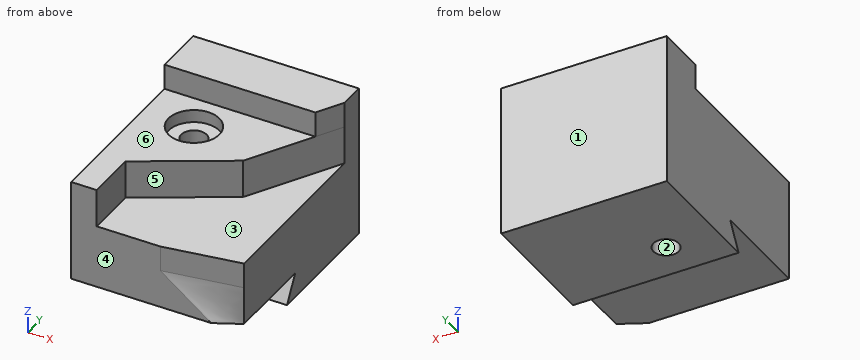
```python
from build123d import *

# Parameters (mm, degrees)
F0_W            = 65
F0_H            = 85
F1_DEPTH        = 25
F3_DEPTH        = 15
F5_DEPTH        = 10
F9_DEPTH        = 10
F12_DEPTH       = 65
F14_D           = 10
F14_CBORE_D     = 20
F14_CBORE_DEPTH = 5


with BuildPart() as f1:
    # F0 (on Top) → F1 (new body)
    with BuildSketch(Plane.XY):
        Rectangle(F0_W, F0_H)
    extrude(amount=F1_DEPTH)

    # F2 (on face) → F3 (join)
    with BuildSketch(Plane.XY.offset(25)):
        Polygon((-32.5, -42.5), (-22.5, -42.5), (-22.5, -22.5), (12.368603, -2.368603), (32.5, 32.5), (32.5, 42.5), (-32.5, 42.5), align=None)
    extrude(amount=F3_DEPTH)

    # F4 (on face) → F5 (join)
    with BuildSketch(Plane.XY.offset(40)):
        Polygon((-32.5, 42.5), (-32.5, 22.5), (26.726497, 22.5), (32.5, 32.5), (32.5, 42.5), align=None)
    extrude(amount=F5_DEPTH)

    # F8 (on face) → F9 (cut)
    with BuildSketch(Plane.XY.offset(25)):
        Polygon((32.5, -37.5), (2.5, -42.5), (32.5, -42.5), align=None)
    extrude(amount=-F9_DEPTH, mode=Mode.SUBTRACT)

    # F9_face (on face) → F10 section 0
    with BuildSketch(Plane(origin=(22.5, -40.833333, 15), x_dir=(1, 0, 0), z_dir=(0, 0, 1))):
        Polygon((10, 3.333333), (-20, -1.666667), (10, -1.666667), align=None)
    # F6 (on face) → F10 section 1
    with BuildSketch(Plane(origin=(0, 0, 0), x_dir=(1, 0, 0), z_dir=(0, 0, -1))):
        Polygon((32.5, 42.5), (22.5, 42.5), (32.5, 37.5), align=None)
    loft(mode=Mode.SUBTRACT)

    # F11 (on face) → F12 (join, through all)
    with BuildSketch(Plane.YZ.offset(32.5)):
        Polygon((42.5, -10), (42.5, 0), (-1.726497, 0), (-7.5, -10), align=None)
    extrude(amount=-F12_DEPTH)

    # F14 (through all)
    with Locations(Plane.XY.offset(40)):
        with Locations((-12.5, 7.5)):
            CounterBoreHole(F14_D / 2, F14_CBORE_D / 2, F14_CBORE_DEPTH)


solid = f1.part
```
Geometry: final body of the model. Coordinates: model frame, mm. Face numbers are marked on the shaded views. A direction names the side the tool comes from. Round coordinates to 2 decimals unless told otherwise and drop trailing zeros. Order: outer loops, then holes, each group sorted by start corner. A loop starts at its lowest first (then second) coordinate and runs counter-clockwise, first axis right, second up. Notation, with made-up numbers: (17, 88) -> (32, 88) arc R18 cw to (32, 119) -> close; hole circle Ø7 at (31, 4). An arc over 180 degrees is marked (long way). Use one line per item in the form item = value.
(1) Section D-D on y = -35. Return loops of the section in (x, z), and give its area (4 significant figures).
Results list:
outline = (-32.5, 0) -> (32.5, 0) -> (32.5, 25) -> (-22.5, 25) -> (-22.5, 40) -> (-32.5, 40) -> close
area = 1,775 mm^2
(2) Access query for the marked faces 4, 5 and 6. Directions: +Z, -Z, +X, -X, +Y, -Y. A direction counts if a zero-diameter tool reaches every point of the face in a straight line with its end or side. Return the directions, or none.
Results list:
face_4 = +Z, -Z, +X, -X, -Y
face_5 = +Z, +X, -Y
face_6 = +Z, +X, -X, -Y
(3) Section C-C on y = 7.5. Return loops of the section in (x, z), and give its area (3 significant figures).
Results list:
outline = (-32.5, -10) -> (-17.5, -10) -> (-17.5, 35) -> (-22.5, 35) -> (-22.5, 40) -> (-32.5, 40) -> close; (-7.5, -10) -> (32.5, -10) -> (32.5, 25) -> (18.07, 25) -> (18.07, 40) -> (-2.5, 40) -> (-2.5, 35) -> (-7.5, 35) -> close
area = 2,480 mm^2
(4) First-contact query: pin 1 Ø1 at (y, z) = (-9, 40) entering from +X; pin 2 Ø12 at (x, y) = (-11, -26.5) entering from +Z; pin 3 Ø19.5 at (x, y) = (5, -13.5) entering from +Z. Flat tips, straight axial feed; report the tip coordinate or a pass-through.
Results list:
pin_1 = 1.75
pin_2 = 25
pin_3 = 40
(5) Draft query along Y for the marked faces 1, 2 and 3. Return one class per face: pulls with the +Y half, pulls with the -Y half, needs draft (parallel to the pull), parting line crosses it, or undercut.
Results list:
face_1 = pulls with the +Y half
face_2 = undercut
face_3 = needs draft
(6) Ray query, probe 1 along Y at (x, z) = (-12.5, 24.5); probe 2 along Z at (x, y) = (29, 19.5); probe 3 along Y at (x, z) = (13.5, 45). Return the intervals inside material, ascending. Write a range as [from, to].
Results list:
probe_1 = [-42.5, 2.5], [12.5, 42.5]
probe_2 = [-10, 25]
probe_3 = [22.5, 42.5]
(7) Section B-B on x = -9.5. Return loops of the section in (y, z), and give its area (3 significant figures).
Results list:
outline = (-42.5, 0) -> (-1.73, 0) -> (-7.5, -10) -> (3.5, -10) -> (3.5, 35) -> (-2.04, 35) -> (-2.04, 40) -> (-14.99, 40) -> (-14.99, 25) -> (-42.5, 25) -> close; (11.5, -10) -> (42.5, -10) -> (42.5, 50) -> (22.5, 50) -> (22.5, 40) -> (17.04, 40) -> (17.04, 35) -> (11.5, 35) -> close
area = 3,200 mm^2
(8) Section A-A on z = 30. Return loops of the section in (x, y).
Results list:
outline = (-32.5, -42.5) -> (-22.5, -42.5) -> (-22.5, -22.5) -> (12.37, -2.37) -> (32.5, 32.5) -> (32.5, 42.5) -> (-32.5, 42.5) -> close; hole circle Ø10 at (-12.5, 7.5)
